Input: dimensioned drawing with shaded views. Units: mm. Origin: part minimum x, y, z. A direction names the side the tool comes from. Give positions to 0.01 mm unless a question says otherwise; leave off trailing zeros. Write each loop counter-clockwise with the first axis right and the second up, starting at its lowest first coordinate (ties: lowest second). Pieces come first, ordered by that corner, then holes. Notation, with made-up numbers: (28, -14.75) -> (77, -14.75) arc R21 ccw to (77, 20.25) -> close; hole circle Ø5 at (89.25, 58.5). An arc over 180 degrees is marked (long way). Return JSON: item names as keys, results as strings. Group by question number.
Item 1: Line query: line 1 (X direction, y = 1.85, z = 13); line 2 (Y direction, x = 9.25, z = 16.5); line 3 (Y direction, x = 13.25, z = 8.25). Output: solid intervals per line, ascending. Write a range as [from, to].
Item 2: Pin query (flat end, axial travel): P1, Ø6, axis at y = 13, z = 7.5, coming from the +X side; P2, Ø4, axis at x = 4.5, y = 9, coming from the +Z side; P3, Ø2, axis at x = 10, y = 11.5, coming from the +Z side; P4, Ø7, axis at y = 8, z = 4.5, coming from the -X side. Return the tip coordinate at first contact, or that it passes through.
Item 3: Mould query, pull axis Y, two halves, no side actions, for the marked faces 6, 7, 8 and 9. Classes: released by +Y, released by -Y, zero draft, split by the parting line, or undercut.
Item 4: Section D-D, the plane z = 9.5. Return loops of the section in (x, y).
Item 5: Section C-C, the plane x = 4. Return loops of the section in (y, z), then the cut area to 3 significant figures.
Item 6: Section A-A, the plane x = 1. Return loops of the section in (y, z).
Item 7: Section B-B, the plane z = 6. Return loops of the section in (x, y).
Item 8: Set-up query: the marked faces 1, 2, 3, 4 and 5. Return all of +Z, -Z, +X, -X, +Y, -Y with unobstructed straight access to the full face (end or side cutting, diameter ignored); none if empty.
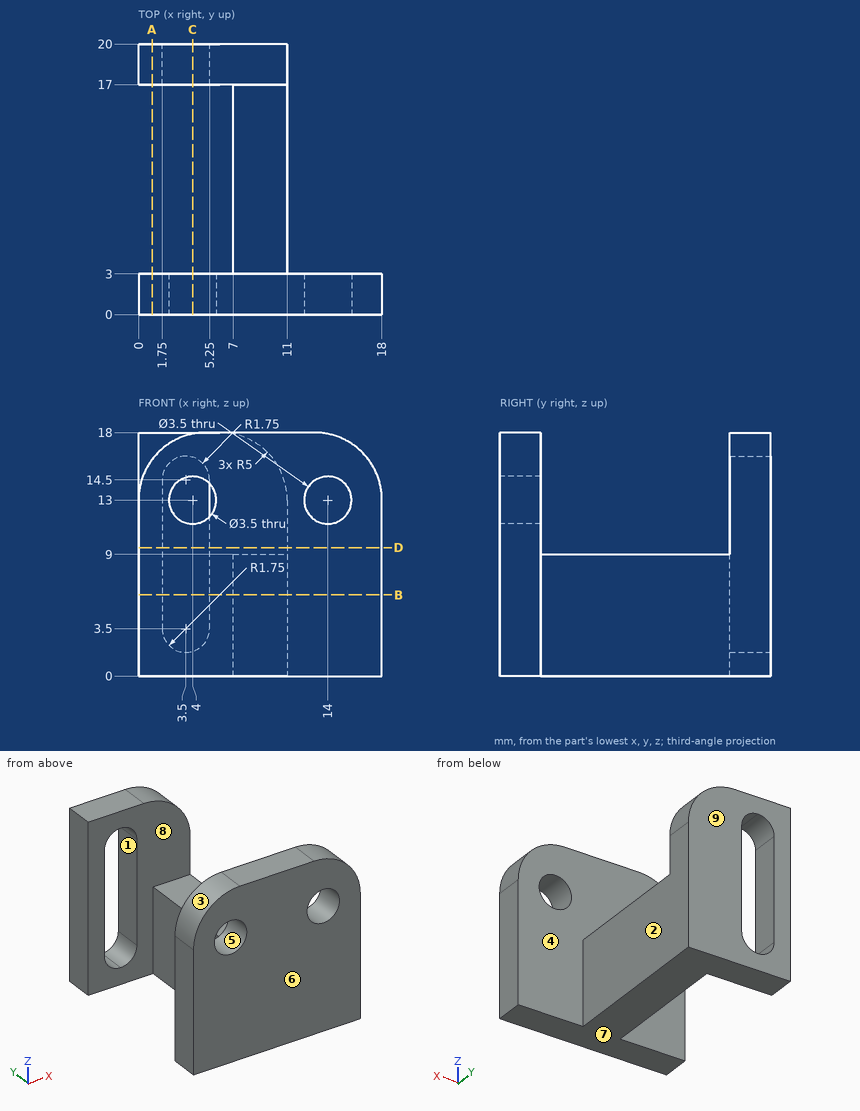
Answer below:
{
 "1": {"line 1": "x = [0, 2.25], [5.75, 12.25], [15.75, 18]", "line 2": "y = [0, 3], [17, 20]", "line 3": "y = [0, 3]"},
 "2": {"P1": "stops at x = 11", "P2": "passes through", "P3": "stops at z = 9", "P4": "stops at x = 7"},
 "3": {"face 6": "released by -Y", "face 7": "zero draft", "face 8": "undercut", "face 9": "released by +Y"},
 "4": {"outline": "(0, 0) -> (18, 0) -> (18, 3) -> (0, 3) -> close; (0, 17) -> (1.75, 17) -> (1.75, 20) -> (0, 20) -> close; (5.25, 17) -> (11, 17) -> (11, 20) -> (5.25, 20) -> close"},
 "5": {"outline": "(0, 0) -> (3, 0) -> (3, 11.25) -> (0, 11.25) -> close; (0, 14.75) -> (3, 14.75) -> (3, 17.9) -> (0, 17.9) -> close; (17, 0) -> (20, 0) -> (20, 1.82) -> (17, 1.82) -> close; (17, 16.18) -> (20, 16.18) -> (20, 18) -> (17, 18) -> close", "area": "54.1 mm2"},
 "6": {"outline": "(0, 0) -> (3, 0) -> (3, 16) -> (0, 16) -> close; (17, 0) -> (20, 0) -> (20, 18) -> (17, 18) -> close"},
 "7": {"outline": "(0, 0) -> (18, 0) -> (18, 3) -> (11, 3) -> (11, 20) -> (5.25, 20) -> (5.25, 17) -> (7, 17) -> (7, 3) -> (0, 3) -> close; (0, 17) -> (1.75, 17) -> (1.75, 20) -> (0, 20) -> close"},
 "8": {"face 1": "+Y", "face 2": "+Z, -Z, +X, +Y", "face 3": "+Z, -X, -Y", "face 4": "+Z", "face 5": "-Y"}
}
